from build123d import *

# Parameters (mm, degrees)
F1_DEPTH = 12.7
F2_W     = 25.4
F2_H     = 254
F3_DEPTH = 254
F4_R     = 5.08


with BuildPart() as f1:
    # F0 (on Front) → F1 (new body, symmetric)
    with BuildSketch(Plane.XZ):
        with BuildLine():
            Line((0, -127), (0, 127))
            ThreePointArc((0, 127), (-127, 0), (0, -127))
        make_face()
    extrude(amount=F1_DEPTH, both=True)

    # F2 (on face) → F3 (join)
    with BuildSketch(Plane.YZ):
        Rectangle(F2_W, F2_H)
    extrude(amount=F3_DEPTH)

    # F4
    f4_edges = [f1.edges().sort_by_distance(p)[0] for p in [
        (127, -12.7, 127),
        (254, -12.7, 0),
    ]]
    fillet(f4_edges, radius=F4_R)


solid = f1.part
Source: CAD feature listing. Evaluate the final solid. Frame: model axes, mm. Coordinates: 2 decimals unless noted, no trailing zeros. Order: outer loops, then holes, each group sorted by start corner. A loop starts at its lowest first (then second) coordinate and runs counter-clockwise, first axis right, second up.
Item 1: First-contact query: P1, Ø3, axis at y = -9, z = -91, coming from the -X side; P2, Ø2, axis at y = 10, z = -77, coming from the -X side; P3, Ø3, axis at x = -39, y = 0.5, coming from the +Z side. Flat tips, straight axial feed; report the tip coordinate or a pass-through.
Output values:
P1: stops at x = -89.92
P2: stops at x = -101.75
P3: stops at z = 121.34
Item 2: Material intervals for line 1 (X direction, y = -5.75, z = 46.5); line 2 (X direction, y = 4.5, z = -71); line 3 (Z direction, x = 107.5, y = -10.5), sorted ascending.
Output values:
line 1: x = -118.18 to 254
line 2: x = -105.3 to 254
line 3: z = -126.1 to 126.1
Item 3: Cut plane A-A (y = -3.5). Return loops of the section in (x, z), plus the area to 3 significant figures.
Output values:
outline: (0, -127) - (254, -127) - (254, 127) - (0, 127) arc R127 ccw to start
area: 89,900 mm2
